The figure shows three views and two pictorial views of one solid part (mm, origin at its lowest corner). Answer the questions. A direction names the side the tool comes from. Round coordinates to 2 decimals unless told otherwise and drop trailing zeros. Write each loop counter-clockwise with the first axis right and the second up, starting at its lowest first coordinate (ties: lowest second). Pieces come first, ordered by that corner, then holes. Notation, with made-up numbers: (31.25, -1) - (57.25, -1) arc R24 ccw to (57.25, 32) - close; hole circle Ø3 at (7.5, 18.5). An arc over 180 degrees is marked (long way). Answer as CSV lines item,"result". Start each with the question number.
Item 1: A cutting plane is placed at A-A on y = 20. Determine the outline of the cut face in (x, z).
Item 2: A cutting plane is placed at C-C on x = 80. Determine the outline of the cut face in (y, z).
Item 3: Which of the six approach directions +Z, -Z, +X, -X, +Y, -Y give full straight-line access (tool end or side, diameter ignored) to the marked faces 1, 2 and 3?
Item 4: For a pull along Y with two mould halves and no side action, classify the marked faces 4, 5 and 6 as pulls with the +Y half, pulls with the -Y half, needs draft (parallel to the pull), parting line crosses it, or undercut.
Item 5: Straight lines are drawn through the part: line 1 along Y through (x, z) = (80, 36.5); line 2 along X through (y, z) = (33, 18); line 3 along Z through (x, y) = (20, 43.5). For each, find the intervals that lie inside material, in ascending order. Write a range as [from, to].
Item 6: Flat-ended cylindrical pins translate along their axes: pin 1 (12 mm diameter, centred on x = 17, z = 26, fed in from -Y); pin 2 (15 mm diameter, centred on x = 54, y = 28.5, fed in from +Z). Find the tip coordinate at first contact, or state that the pin passes through.
Item 7: A cutting plane is placed at B-B on z = 39.5. Determine the outline of the cut face in (x, y), and give its area (3 significant figures).
Item 8: A cutting plane is placed at D-D on z = 14.5. Determine the outline of the cut face in (x, y).
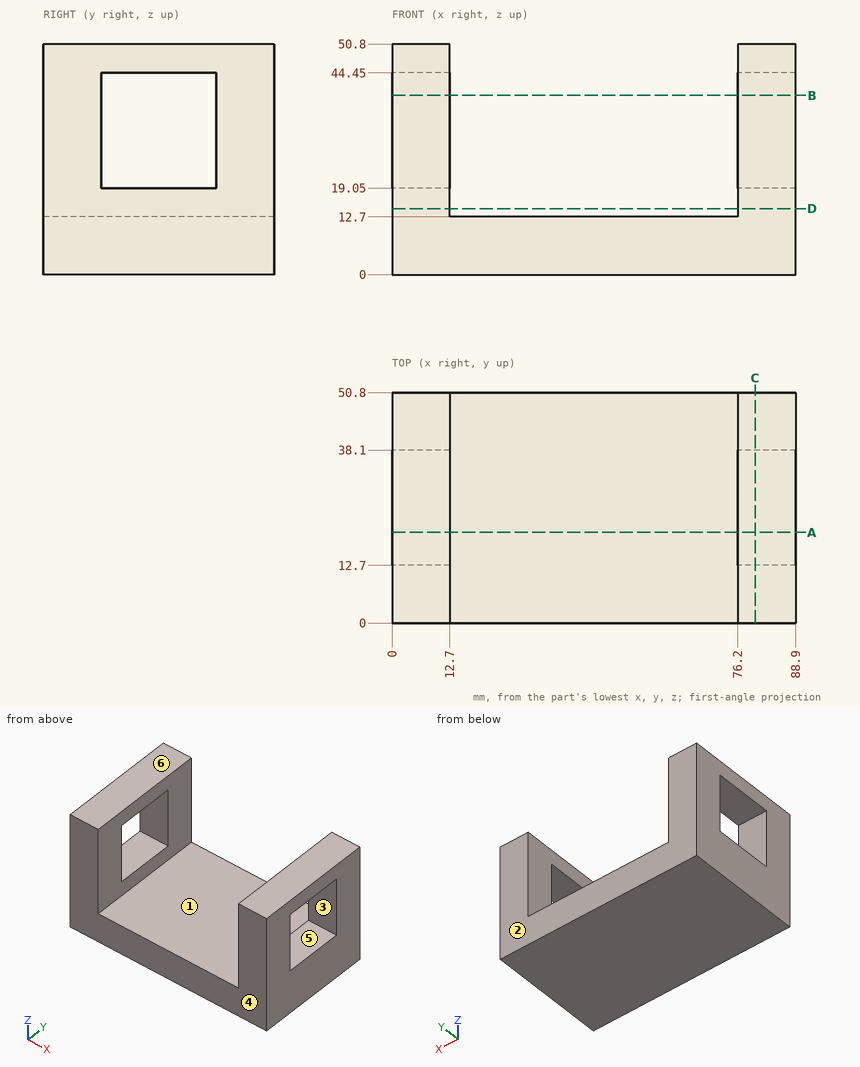
Geometry says:
1,outline,"(0, 0) - (88.9, 0) - (88.9, 19.05) - (76.2, 19.05) - (76.2, 12.7) - (12.7, 12.7) - (12.7, 19.05) - (0, 19.05) - close; (0, 44.45) - (12.7, 44.45) - (12.7, 50.8) - (0, 50.8) - close; (76.2, 44.45) - (88.9, 44.45) - (88.9, 50.8) - (76.2, 50.8) - close"
2,outline,"(0, 0) - (50.8, 0) - (50.8, 50.8) - (0, 50.8) - close; hole (12.7, 19.05) - (38.1, 19.05) - (38.1, 44.45) - (12.7, 44.45) - close"
3,face 1,"+Z, +Y, -Y"
3,face 2,"+Z, -Z, +X, -X, +Y"
3,face 3,"+X, -X"
4,face 4,"pulls with the -Y half"
4,face 5,"undercut"
4,face 6,"needs draft"
5,line 1,"y = [0, 12.7], [38.1, 50.8]"
5,line 2,"x = [0, 12.7], [76.2, 88.9]"
5,line 3,"z = [0, 12.7]"
6,pin 1,"stops at y = 0"
6,pin 2,"stops at z = 12.7"
7,outline,"(0, 0) - (12.7, 0) - (12.7, 12.7) - (0, 12.7) - close; (0, 38.1) - (12.7, 38.1) - (12.7, 50.8) - (0, 50.8) - close; (76.2, 0) - (88.9, 0) - (88.9, 12.7) - (76.2, 12.7) - close; (76.2, 38.1) - (88.9, 38.1) - (88.9, 50.8) - (76.2, 50.8) - close"
7,area,"645 mm^2"
8,outline,"(0, 0) - (12.7, 0) - (12.7, 50.8) - (0, 50.8) - close; (76.2, 0) - (88.9, 0) - (88.9, 50.8) - (76.2, 50.8) - close"
